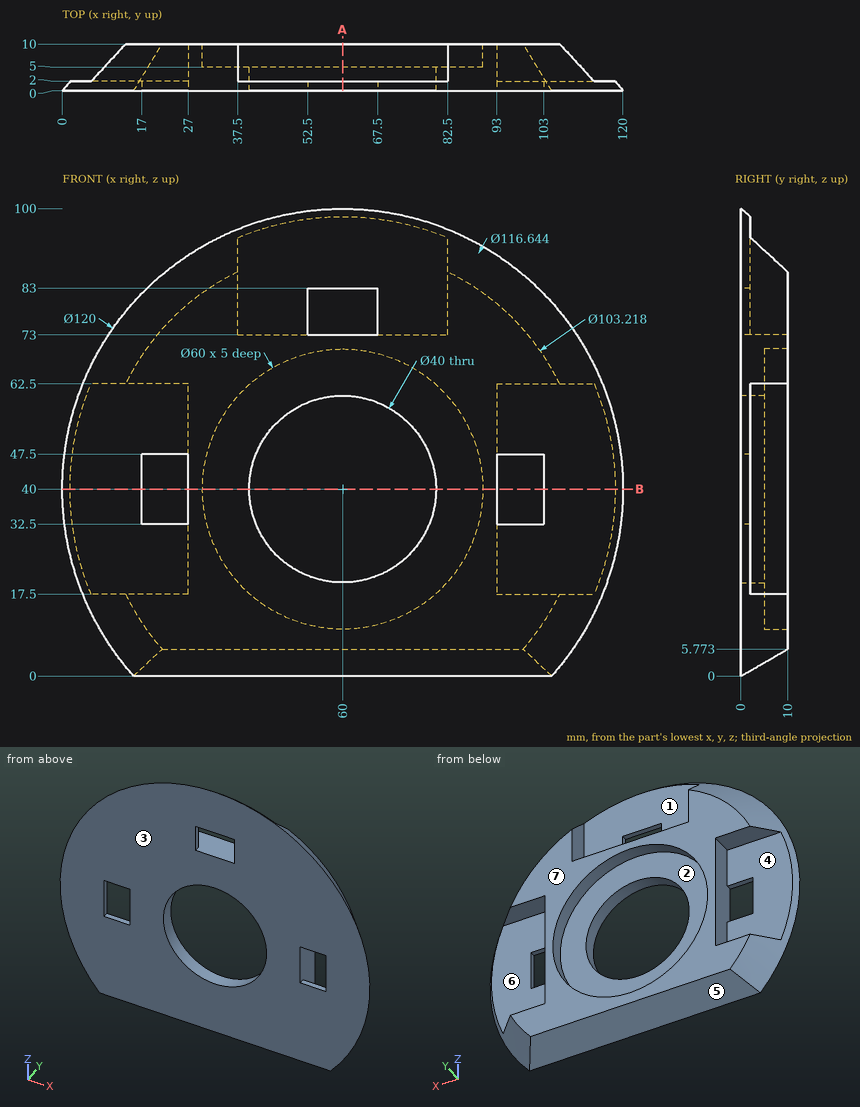
Check sheet for the drawn part. Datum: minimum x, y, z corner. Units: mm. A direction names the side the tool comes from. Coordinates: 2 decimals unless noted, no trailing zeros. Order: outer loops, then holes, each group sorted by start corner. A loop starts at its lowest first (then second) coordinate and runs counter-clockwise, first axis right, second up. Notation, with made-up numbers: (11, 20) -> (65, 20) arc R17 ccw to (65, 49) -> close; hole circle Ø2 at (84, 79.5). An arc over 180 degrees is marked (long way). Use a Markdown table: item, result. Add a question column.
1. Go/stop test with flat-tipped pins: pin 1 Ø2 at (y, z) = (1, 76.5) entering from -X (1 decimal); pin 2 Ø1 at (y, z) = (0.5, 78.5) entering from +X; pin 3 Ø12.5 at (x, z) = (50, 91.5) entering from +Y; pin 4 Ø4 at (x, z) = (100.5, 39.5) entering from +Y. Record where each tip stops, or that it passes through.
2. Cross-section at B-B (z = 40). Enter the section's corners in (x, y).
3. Set-up check for the marked faces 1, 2, 3 and 4: record each of +Z, -Z, +X, -X, +Y, -Y from which the full face is reachable in a straight line by a thin tool's end or side.
4. Mould release check, pull along Z, two halves, no side actions. Record for the marked faces 5, 6 and 7: pulls with the +Z half, pulls with the -Z half, needs draft (parallel to the pull), parting line crosses it, or undercut.
5. Cross-section at A-A (x = 60). Give the number of separate pieces and of enclosed holes in the cut face.
6. Material ranges on L1, parallel to X at y = 2.7, z = 40; L2, parallel to X at y = 6.45, z = 40; L3, parallel to Y at x = 106, z = 34, recorded low to high.
Filled sheet:
| question | item | result |
|---|---|---|
| 1 | pin 1 | x = 12.1 |
| 1 | pin 2 | x = 106.16 |
| 1 | pin 3 | y = 2 |
| 1 | pin 4 | through |
| 2 | outline | (0, 0) -> (17, 0) -> (17, 2) -> (1.68, 2) -> close; (27, 0) -> (40, 0) -> (40, 5) -> (30, 5) -> (30, 10) -> (27, 10) -> close; (80, 0) -> (93, 0) -> (93, 10) -> (90, 10) -> (90, 5) -> (80, 5) -> close; (103, 0) -> (120, 0) -> (118.32, 2) -> (103, 2) -> close |
| 3 | face 1 | +Z, +Y |
| 3 | face 2 | +Y |
| 3 | face 3 | +Z, -Z, +X, -X, -Y |
| 3 | face 4 | -X, +Y |
| 4 | face 5 | pulls with the -Z half |
| 4 | face 6 | undercut |
| 4 | face 7 | needs draft |
| 5 | separate pieces | 3 |
| 5 | enclosed holes | 0 |
| 6 | L1 | 27 to 40, 80 to 93 |
| 6 | L2 | 27 to 30, 90 to 93 |
| 6 | L3 | 0 to 2 |
